Geometry check sheet. Reference: the model listing, model coordinates, mm. Coordinates: 2 decimals unless noted, no trailing zeros. Order: outer loops, then holes, each group sorted by start corner. A loop starts at its lowest first (then second) coordinate and runs counter-clockwise, first axis right, second up. Notation, with made-up numbers: (71.5, 9.25) - (96.5, 9.25) arc R26 ccw to (96.5, 42.25) - close; hole circle Ø10 at (-3.5, 14). An arc over 180 degrees is marked (long way). Return JSON: item names as keys, results as strings. Group by question number.
Item 1: Section check D-D on x = 69.5. Enter the section's corners in (y, z), then the cut area to 3 significant figures.
Item 2: Section check C-C on x = -33. Enter the section's corners in (y, z), then the cut area to 3 significant figures.
Item 3: Gauge pin test, flat ends, axial feed: pin 1 (12 mm diameter, centred on x = -46.5, y = -18.5, fed in from +Z); pin 2 (4 mm diameter, centred on x = 67.5, z = 6.5, fed in from +Y). Record the tip position at first contact, or that the pin passes through.
Item 4: Section check B-B on z = 4.25. Enter the section's corners in (x, y).
Item 5: Scan lines: probe 1 along Y at (x, z) = (-25, 5.5); probe 2 along X at (y, z) = (-13.5, 2); probe 3 along Y at (x, z) = (72, 3.75). Record each from-to range of solid material in increasing order.
Item 6: Section check A-A on y = 0. Enter the section's corners in (x, z).
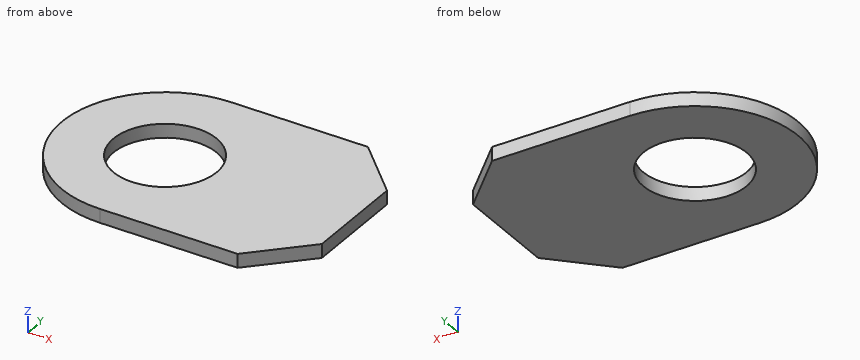
Autodesk Inventor part; units mm, degrees
ref_plane "YZ Plane" through (0, 0, 0) normal (1, 0, 0) x (0, 1, 0)
ref_plane "XZ Plane" through (0, 0, 0) normal (0, 1, 0) x (-1, 0, 0)
ref_plane "XY Plane" through (0, 0, 0) normal (0, 0, 1) x (1, 0, 0)
sketch "Sketch1" plane through (0, 0, 0) normal (0, 0, 1) x (1, 0, 0)
  line L0 (-85, 60) -> (85, 60)
  line L1 (85, 60) -> (85, -60)
  line L2 (85, -60) -> (-85, -60)
  line L3 (-85, -60) -> (-85, 60)
  line L4 (-85, 60) -> (85, -60) construction
  line L5 (85, 60) -> (-85, -60) construction
  circle A0 centre (-25, 0) radius 30
  line L6 (0, 60) -> (0, -60) construction
  arc A1 (-25, 60) -> (-25, -60) centre (-25, 0) ccw
  line L7 (55, 60) -> (85, 30)
  line L8 (85, -30) -> (55, -60)
  point P0 (0, 0)
  point P1 (-85, 0)
  dimension "d0" = 170
  dimension "d1" = 120
  dimension "d13" = 60
  dimension "d14" = 60
  dimension "d15" = 30
  dimension "d17" = 45
extrude "Plate1" add sketch "Sketch1" along normal blind 8 contours L0 L7 L1 L8 L2 A1
equation "\"d2\" = Thickness"
equation "\"BendRadius\" = Thickness"
equation "\"BendReliefWidth\" = Thickness"
equation "\"BendReliefDepth\" = 0.5 * Thickness"
equation "\"CornerReliefSize\" = 4 * Thickness"
equation "\"MinimumRemnant\" = 2 * Thickness"
equation "\"TransitionRadius\" = BendRadius"
equation "\"JacobiRadiusSize\" = BendRadius"
equation "\"GapSize\" = Thickness"
properties part number "ухо"
Computed:
{
 "1": {"outline": "(-45.5, 0) - (45.5, 0) - (45.5, 8) - (-45.5, 8) - close", "area": "728 mm²"},
 "2": {"outline": "(-59.46, 0) - (-28.91, 0) - (-28.91, 8) - (-59.46, 8) - close; (28.91, 0) - (59.46, 0) - (59.46, 8) - (28.91, 8) - close", "area": "489 mm²"},
 "3": {"pin 1": "stops at z = 8", "pin 2": "stops at y = 49.5"},
 "4": {"outline": "(-25, -60) - (55, -60) - (85, -30) - (85, 30) - (55, 60) - (-25, 60) arc R60 ccw to start; hole circle Ø60 at (-25, 0)"},
 "5": {"probe 1": "y = -60 to -30, 30 to 60", "probe 2": "x = -83.46 to -51.79, 1.79 to 85", "probe 3": "y = -43 to 43"},
 "6": {"outline": "(-85, 0) - (-55, 0) - (-55, 8) - (-85, 8) - close; (5, 0) - (85, 0) - (85, 8) - (5, 8) - close"}
}
